The model under review builds one solid part; all positions refer to its coordinate system, in mm. A direction names the side the tool comes from. Give positions to 0.01 mm unless a question says otherwise; leave off trailing zeros. Loops run counter-clockwise (first coordinate to the right, second up) from the corner with the lowest first, then second, coordinate; pieces in that order, holes last. Notation, with made-up numbers: M 34.25,-35.75 L 87.25,-35.75 A33 cw 87.25,-6.75 Z; hole C -37.75,-31 d6. An arc over 180 degrees is marked long. Write item = value, one per line. Start each with the question number.
1. We need section C-C on x = 15.5. Give the boundary of the cut face in (y, z).
2. Wall thickness on line 1 along Z through (x, y) = (7.25, 10.5); line 2 along Y through (x, z) = (12.5, 8.75); line 3 along X through (y, z) = (16.5, 5.5): over which ranges is each line inside the solid? List them lowest first. Write a range as from..to.
3. We need section B-B on y = 8.5. Give the boundary of the cut face in (x, z), then the cut area to 3 significant figures.
4. We need section A-A on z = 8.75. Give the boundary of the cut face in (x, y), then the cut area to 3 significant figures.
5. We need section D-D on y = 17. Give the boundary of the cut face in (x, z).
6. For pin 1 (2 mm diameter, centred on x = 12, z = 6.5, fed in from +Y); pin 2 (3 mm diameter, centred on y = 15, z = 11.5, fed in from -X); pin 3 (0.9 mm diameter, centred on x = 1.5, z = 11.5, fed in from +Y), all flat-tipped, find the tip position at first contact; note any pin that passes through.
7. For faces 1 (the face through (3, 10, 1)), 2 (the face through (10, 17, 10)), 3 (the face through (5.4, 12.4, 12.85)), list the 3-axis set-ups (+Z, -Z, +X, -X, +Y, -Y) from which the entire face can be reached by the end or side of a thin tool; tool diameter is ignored.
8. Draft analysis for pull direction Y (two halves, no side actions). For faces 4 (the face through (8, 20, 10)), 5 (the face through (14.839, 11.168, 9.86)), 6 (the face through (5, 15, 19)), state which applies: pulls with the +Y half, pulls with the -Y half, needs draft (parallel to the pull), parting line crosses it, or undercut.
from build123d import *

# Parameters (mm, degrees)
SKETCH1_R           = 4.35
BOSS_EXTRUDE1_DEPTH = 20
SKETCH2_W           = 7.5
SKETCH2_H           = 1.8
SKETCH2_H_2         = 2.5
SKETCH2_H_3         = 4.3
CUT_EXTRUDE1_DEPTH  = 12.5


with BuildPart() as part:
    # Sketch1 → Boss-Extrude1 (new body)
    with BuildSketch(Plane.XY):
        with BuildLine():
            Line((0, 0), (20, 0))
            Line((20, 0), (20, 7.5))
            ThreePointArc((20, 7.5), (17.803300859, 12.803300859), (12.5, 15))
            Line((12.5, 15), (10, 15))
            Line((10, 15), (10, 20))
            Line((10, 20), (5, 20))
            Line((5, 20), (5, 10))
            Line((5, 10), (0, 10))
            Line((0, 10), (0, 0))
        make_face()
        with Locations((12.5, 7.5)):
            Circle(SKETCH1_R, mode=Mode.SUBTRACT)
    extrude(amount=BOSS_EXTRUDE1_DEPTH)

    # Sketch2 → Cut-Extrude1 (cut)
    with BuildSketch(Plane(origin=(0, 20, 0), x_dir=(1, 0, 0), z_dir=(0, 1, 0))):
        with Locations((3.75, -3.75)):
            Rectangle(SKETCH2_W, SKETCH2_H)
        with Locations((3.75, -8.75)):
            Rectangle(SKETCH2_W, SKETCH2_H_2)
        with Locations((3.75, -15)):
            Rectangle(SKETCH2_W, SKETCH2_H_3)
    extrude(amount=-CUT_EXTRUDE1_DEPTH, mode=Mode.SUBTRACT)


solid = part.part
Final values:
q1.outline = M 0,0 L 4.35,0 L 4.35,20 L 0,20 Z; M 10.65,0 L 14.37,0 L 14.37,20 L 10.65,20 Z
q2.line_1 = 0..2.85, 4.65..7.5, 10..12.85, 17.15..20
q2.line_2 = 0..3.15, 11.85..15
q2.line_3 = 5..10
q3.outline = M 0,0 L 8.27,0 L 8.27,20 L 0,20 L 0,17.15 L 7.5,17.15 L 7.5,12.85 L 0,12.85 L 0,10 L 7.5,10 L 7.5,7.5 L 0,7.5 L 0,4.65 L 7.5,4.65 L 7.5,2.85 L 0,2.85 Z; M 16.73,0 L 19.93,0 L 19.93,20 L 16.73,20 Z
q3.area = 165 mm²
q4.outline = M 0,0 L 20,0 L 20,7.5 A7.5 ccw 12.5,15 L 10,15 L 10,20 L 7.5,20 L 7.5,7.5 L 0,7.5 Z; hole C 12.5,7.5 d8.7
q4.area = 185 mm²
q5.outline = M 5,0 L 10,0 L 10,20 L 5,20 L 5,17.15 L 7.5,17.15 L 7.5,12.85 L 5,12.85 L 5,10 L 7.5,10 L 7.5,7.5 L 5,7.5 L 5,4.65 L 7.5,4.65 L 7.5,2.85 L 5,2.85 Z
q6.pin_1 = 15
q6.pin_2 = 5
q6.pin_3 = 10
q7.face_1 = +Z, -Z, -X, +Y
q7.face_2 = +Z, -Z, +X, +Y
q7.face_3 = -X, +Y
q8.face_4 = pulls with the +Y half
q8.face_5 = undercut
q8.face_6 = needs draft
